The listing builds one solid part. Answer for the finished solid, in the listing's coordinates (mm). Round coordinates to 2 decimals unless told otherwise and drop trailing zeros. Loops run counter-clockwise (first coordinate to the right, second up) from the corner with the lowest first, then second, coordinate; pieces in that order, holes last. Notation, with made-up numbers: (-19.75, 11) -> (-2.75, 11) arc R20 ccw to (-2.75, 39) -> close; hole circle Ø9 at (65.5, 77.5). An arc over 180 degrees is marked (long way). Answer in a Markdown table with one row per item. Add a question column.
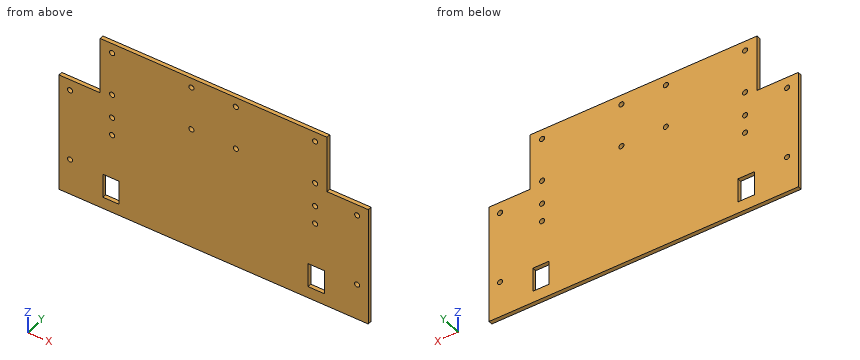
```python
from build123d import *

# Parameters (mm, degrees)
CROQUIS1_R              = 1.625
CUERPO_INICIAL_DEPTH    = 2.5
SALIENTE_EXTRUIR2_DEPTH = 195
CROQUIS7_R              = 1.625
CORTAR_EXTRUIR2_DEPTH   = 10
CROQUIS10_R             = 1.625
CORTAR_EXTRUIR7_DEPTH   = 10
CROQUIS11_W             = 10.25
CROQUIS11_H             = 15.25
CORTAR_EXTRUIR8_DEPTH   = 10
SALIENTE_EXTRUIR3_DEPTH = 195


with BuildPart() as part:
    # Croquis1 → Cuerpo Inicial (new body)
    with BuildSketch(Plane(origin=(0, 0, 0), x_dir=(1, 0, 0), z_dir=(0, 1, 0))):
        Polygon((-71.5, -25), (-71.5, -61), (71.5, -61), (71.5, -25), (97.5, -25), (97.5, 0), (97.5, 1), (97.5, 5.7), (45, 5.7), (-45, 5.7), (-97.5, 5.7), (-97.5, 1), (-97.5, 0), (-97.5, -25), align=None)
        with Locations(Location((-90.5, -18, 0), (0, 0, 270))):
            Circle(CROQUIS1_R, mode=Mode.SUBTRACT)
        with Locations(Location((90.5, -18, 0), (0, 0, 270))):
            Circle(CROQUIS1_R, mode=Mode.SUBTRACT)
    extrude(amount=CUERPO_INICIAL_DEPTH)

    # Croquis3 → Saliente-Extruir2 (add)
    with BuildSketch(Plane(origin=(97.5, 0, 0), x_dir=(0, 0, -1), z_dir=(1, 0, 0))):
        Polygon((5.7, 2.5), (47.783199952, 2.5), (50.7, 0), (5.7, 0), align=None)
    extrude(amount=-SALIENTE_EXTRUIR2_DEPTH)

    # Croquis7 → Cortar-Extruir2 (cut)
    with BuildSketch(Plane(origin=(0, 2.5, 0), x_dir=(1, 0, 0), z_dir=(0, 1, 0))):
        with Locations(Location((90.5, 27.783199952, 0), (0, 0, 270))):
            Circle(CROQUIS7_R)
        with Locations(Location((-90.5, 27.783199952, 0), (0, 0, 270))):
            Circle(CROQUIS7_R)
    extrude(amount=-CORTAR_EXTRUIR2_DEPTH, mode=Mode.SUBTRACT)

    # Croquis10 → Cortar-Extruir7 (cut)
    with BuildSketch(Plane(origin=(0, 2.5, -2.5), x_dir=(1, 0, 0), z_dir=(0, -1, 0))):
        with Locations(Location((64, 2.96, 0), (0, 0, 90))):
            Circle(CROQUIS10_R)
        with Locations(Location((64, 14.5, 0), (0, 0, 90))):
            Circle(CROQUIS10_R)
        with Locations(Location((-64, 2.96, 0), (0, 0, 90))):
            Circle(CROQUIS10_R)
        with Locations(Location((-64, 14.5, 0), (0, 0, 90))):
            Circle(CROQUIS10_R)
        with Locations(Location((64, 29.6754, 0), (0, 0, 90))):
            Circle(CROQUIS10_R)
        with Locations(Location((64, 57.3245, 0), (0, 0, 90))):
            Circle(CROQUIS10_R)
        with Locations(Location((-64, 57.3245, 0), (0, 0, 90))):
            Circle(CROQUIS10_R)
        with Locations(Location((-64, 29.6754, 0), (0, 0, 90))):
            Circle(CROQUIS10_R)
        with Locations(Location((14, 29.6754, 0), (0, 0, 90))):
            Circle(CROQUIS10_R)
        with Locations(Location((14, 57.3245, 0), (0, 0, 90))):
            Circle(CROQUIS10_R)
        with Locations(Location((-14, 57.3245, 0), (0, 0, 90))):
            Circle(CROQUIS10_R)
        with Locations(Location((-14, 29.6754, 0), (0, 0, 90))):
            Circle(CROQUIS10_R)
    extrude(amount=CORTAR_EXTRUIR7_DEPTH, mode=Mode.SUBTRACT)

    # Croquis11 → Cortar-Extruir8 (cut)
    with BuildSketch(Plane.XZ):
        with Locations((-64.64307361, -35.7)):
            Rectangle(CROQUIS11_W, CROQUIS11_H)
        with Locations((64.64307361, -35.7)):
            Rectangle(CROQUIS11_W, CROQUIS11_H)
    extrude(amount=-CORTAR_EXTRUIR8_DEPTH, mode=Mode.SUBTRACT)

    # Croquis12 → Saliente-Extruir3 (add)
    with BuildSketch(Plane.ZY.offset(97.5)):
        Polygon((-50.7, 0), (-47.783199952, 2.5), (-50.7, 2.5), align=None)
    extrude(amount=-SALIENTE_EXTRUIR3_DEPTH)


solid = part.part
```
Item 1: Section C-C, the plane x = -81 is taken. Write down the section's boundary in (y, z), and give its area (3 significant figures).
Item 2: Section A-A, the plane y = 1 is taken. Give the number of separate pieces and of enclosed holes in the cut face, and give its area (3 significant figures).
Item 3: Section B-B, the plane z = -39.5 is taken. Write down the section's boundary in (x, y), and give its area (3 significant figures).
Item 4: Consider L1, parallel to X at y = 0.65, z = 12 (3 decimals); L2, parallel to Z at x = -14, y = 1.6; L3, parallel to Z at x = 64, y = 1.3 (1 decimal). Determine where each line is inside the solid, lowest interval first. Write a range as from..to.
Item 5: Section D-D, the plane z = 40.5 is taken. Write down the section's boundary in (x, y), and give its area (4 significant figures).
Item 6: Flat-ended cylindrical pins translate along their axes: P1, Ø1.2, axis at y = 2, z = 34.5, coming from the -X side; P2, Ø2.5, axis at x = -64, z = 0.46, coming from the -Y side; P3, Ø0.8, axis at x = 89.5, y = 0.5, coming from the +Z side. Find the tip coordinate at first contact, or state that the pin passes through.
Here are the results:
| question | item | result |
|---|---|---|
| 1 | outline | (0, -50.7) -> (2.5, -50.7) -> (2.5, 25) -> (0, 25) -> close |
| 1 | area | 189 mm² |
| 2 | separate pieces | 1 |
| 2 | enclosed holes | 18 |
| 2 | area | 19,500 mm² |
| 3 | outline | (-97.5, 0) -> (-69.77, 0) -> (-69.77, 2.5) -> (-97.5, 2.5) -> close; (-59.52, 0) -> (59.52, 0) -> (59.52, 2.5) -> (-59.52, 2.5) -> close; (69.77, 0) -> (97.5, 0) -> (97.5, 2.5) -> (69.77, 2.5) -> close |
| 3 | area | 436 mm² |
| 4 | L1 | x = -97.5..-65.625, -62.375..62.375, 65.625..97.5 |
| 4 | L2 | z = -50.7..25.55, 28.8..53.2, 56.45..61 |
| 4 | L3 | z = -50.7..-43.3, -28.1..-1.2, 2.1..10.4, 13.6..25.6, 28.8..53.2, 56.4..61 |
| 5 | outline | (-71.5, 0) -> (71.5, 0) -> (71.5, 2.5) -> (-71.5, 2.5) -> close |
| 5 | area | 357.5 mm² |
| 6 | P1 | stops at x = -71.5 |
| 6 | P2 | passes through |
| 6 | P3 | stops at z = 25 |
